Check sheet for the modelled part. Datum: model origin and axes. Units: mm. A direction names the side the tool comes from. Coordinates: 2 decimals unless noted, no trailing zeros. Loops run counter-clockwise (first coordinate to the right, second up) from the corner with the lowest first, then second, coordinate; pieces in that order, holes last. Notation, with made-up numbers: (44.25, -33) - (92.25, -33) arc R26 cw to (92.25, -13) - close; hole circle Ø6 at (24.5, 82). An arc over 180 degrees is marked (long way). Answer as a JSON object with one key per item and string values. Group by question number.
from build123d import *

# Parameters (mm, degrees)
SKETCH1_W           = 45
SKETCH1_H           = 10
BOSS_EXTRUDE1_DEPTH = 10
SKETCH2_W           = 10
SKETCH2_H           = 5
SKETCH2_W_2         = 12
BOSS_EXTRUDE2_DEPTH = 10
SKETCH3_W           = 10
SKETCH3_H           = 5
BOSS_EXTRUDE3_DEPTH = 10
SKETCH4_R           = 1.5
CUT_EXTRUDE1_DEPTH  = 5
SKETCH6_R           = 1.5
CUT_EXTRUDE3_DEPTH  = 5
CUT_EXTRUDE4_START  = -5
SKETCH7_R           = 1.5
CUT_EXTRUDE4_DEPTH  = 5
SKETCH9_R           = 1.5
CUT_EXTRUDE6_DEPTH  = 5
SKETCH10_R          = 1.5
CUT_EXTRUDE7_DEPTH  = 5
SKETCH11_W          = 12
SKETCH11_H          = 5.7
BOSS_EXTRUDE4_DEPTH = 2.7


with BuildPart() as part:
    # Sketch1 → Boss-Extrude1 (new body)
    with BuildSketch(Plane.XY):
        with Locations((22.5, 5)):
            Rectangle(SKETCH1_W, SKETCH1_H)
    extrude(amount=BOSS_EXTRUDE1_DEPTH)

    # Sketch2 → Boss-Extrude2 (add)
    with BuildSketch(Plane(origin=(0, 10, 0), x_dir=(1, 0, 0), z_dir=(0, 1, 0))):
        with Locations((40, -2.5)):
            Rectangle(SKETCH2_W, SKETCH2_H)
        with Locations((12.3, -2.5)):
            Rectangle(SKETCH2_W_2, SKETCH2_H)
    extrude(amount=BOSS_EXTRUDE2_DEPTH)

    # Sketch3 → Boss-Extrude3 (add)
    with BuildSketch(Plane.XY.offset(10)):
        with Locations((5, 2.5)):
            Rectangle(SKETCH3_W, SKETCH3_H)
        with Locations((40, 2.5)):
            Rectangle(SKETCH3_W, SKETCH3_H)
    extrude(amount=BOSS_EXTRUDE3_DEPTH)

    # Sketch4 → Cut-Extrude1 (cut)
    with BuildSketch(Plane.ZY):
        with Locations((5, 5)):
            Circle(SKETCH4_R)
    extrude(amount=-CUT_EXTRUDE1_DEPTH, mode=Mode.SUBTRACT)

    # Sketch6 → Cut-Extrude3 (cut)
    with BuildSketch(Plane(origin=(0, 5, 0), x_dir=(1, 0, 0), z_dir=(0, 1, 0))):
        with Locations(Location((5, -15, 0), (0, 0, 270))):
            Circle(SKETCH6_R)
    extrude(amount=-CUT_EXTRUDE3_DEPTH, mode=Mode.SUBTRACT)

    # Sketch7 → Cut-Extrude4 (cut)
    with BuildSketch(Plane(origin=(45, 0, 0), x_dir=(0, 0, -1), z_dir=(1, 0, 0)).offset(CUT_EXTRUDE4_START)):
        with Locations(Location((-5, 5, 0), (0, 0, 180))):
            Circle(SKETCH7_R)
    extrude(amount=CUT_EXTRUDE4_DEPTH, mode=Mode.SUBTRACT)

    # Sketch9 → Cut-Extrude6 (cut)
    with BuildSketch(Plane(origin=(0, 5, 0), x_dir=(1, 0, 0), z_dir=(0, 1, 0))):
        with Locations(Location((40, -15, 0), (0, 0, 180))):
            Circle(SKETCH9_R)
    extrude(amount=-CUT_EXTRUDE6_DEPTH, mode=Mode.SUBTRACT)

    # Sketch10 → Cut-Extrude7 (cut)
    with BuildSketch(Plane.XY.offset(5)):
        with Locations((40, 15)):
            Circle(SKETCH10_R)
    extrude(amount=-CUT_EXTRUDE7_DEPTH, mode=Mode.SUBTRACT)

    # Sketch11 → Boss-Extrude4 (add)
    with BuildSketch(Plane(origin=(0, 0, 0), x_dir=(-1, 0, 0), z_dir=(0, 0, -1))):
        with Locations((-12.3, 17.15)):
            Rectangle(SKETCH11_W, SKETCH11_H)
    extrude(amount=BOSS_EXTRUDE4_DEPTH)


solid = part.part
1. Gauge pin test, flat ends, axial feed: pin 1 (1.5 mm diameter, centred on y = 13.5, z = 2.5, fed in from -X); pin 2 (12 mm diameter, centred on x = 30.5, z = 10, fed in from +Y); pin 3 (5.5 mm diameter, centred on y = 2, z = 16.5, fed in from -X); pin 4 (2 mm diameter, centred on x = 22, y = 2, fed in from +Z). Record the tip position at first contact, or that the pin passes through.
2. Release check for a two-part mould opening along X. For faces 4 (the face through (35, 15, 3)), 5 (the face through (12, 17, -2.7)), 6 (the face through (5, 5, 5)) record: released by +X, released by -X, zero draft, split by the parting line, or undercut.
3. Sectioned sample at A-A on y = 15. Record the cut outline in (x, z), plus the area to 3 significant figures.
4. Access from +Z, -Z, +X, -X, +Y, -Y to the whole of each face (thin tool, end or side, straight path). Record for faces 1 (the face through (38.8, 5, 13.8)), 2 (the face through (10, 2, 15)), 3 (the face through (42.46, 4.55, 6.43)).
5. Material ranges on line 1 (X direction, y = 10.5, z = 4.25); line 2 (Z direction, x = 40, y = 3.2); line 3 (Y direction, x = 4.5, z = 5), recorded low to high.
6. Sectioned sample at D-D on y = 1.5. Record the cut outline in (x, z), plus the area to 3 significant figures.
7. Sectioned sample at B-B on z = 15. Record the cut outline in (x, y).
8. Sectioned sample at C-C on y = 11.5. Record the cut outline in (x, z).
Answers follow:
{
 "1": {"pin 1": "stops at x = 6.3", "pin 2": "stops at y = 10", "pin 3": "stops at x = 0", "pin 4": "stops at z = 10"},
 "2": {"face 4": "undercut", "face 5": "zero draft", "face 6": "released by -X"},
 "3": {"outline": "(6.3, -2.7) - (18.3, -2.7) - (18.3, 5) - (6.3, 5) - close; (35, 0) - (38.5, 0) - (38.5, 5) - (35, 5) - close; (41.5, 0) - (45, 0) - (45, 5) - (41.5, 5) - close", "area": "127 mm^2"},
 "4": {"face 1": "+Z, +X, -X, +Y", "face 2": "+Z, +Y, -Y", "face 3": "+X"},
 "5": {"line 1": "x = 6.3 to 18.3, 35 to 45", "line 2": "z = 0 to 13.5, 16.5 to 20", "line 3": "y = 0 to 3.5, 6.5 to 10"},
 "6": {"outline": "(0, 0) - (45, 0) - (45, 20) - (35, 20) - (35, 10) - (10, 10) - (10, 20) - (0, 20) - close; hole circle Ø3 at (5, 15); hole circle Ø3 at (40, 15)", "area": "636 mm^2"},
 "7": {"outline": "(0, 0) - (3.5, 0) - (3.5, 5) - (0, 5) - close; (6.5, 0) - (10, 0) - (10, 5) - (6.5, 5) - close; (35, 0) - (38.5, 0) - (38.5, 5) - (35, 5) - close; (41.5, 0) - (45, 0) - (45, 5) - (41.5, 5) - close"},
 "8": {"outline": "(6.3, 0) - (18.3, 0) - (18.3, 5) - (6.3, 5) - close; (35, 0) - (45, 0) - (45, 5) - (35, 5) - close"}
}
